Geometry check sheet. Reference: the model listing, model coordinates, mm. A direction names the side the tool comes from. Round coordinates to 2 decimals unless told otherwise and drop trailing zeros. Write item = value, one per line.
from build123d import *

# Parameters (mm, degrees)
SKETCH_1_R               = 1.75
EXTRUDE_1_DEPTH          = 6.6
EXTRUDE_1_2_DEPTH        = 6.6
SKETCH_2_R               = 50
EXTRUDE_2_DEPTH          = 3.4
SKETCH_4_R               = 1.75
CUT_EXTRUDE_2_DEPTH      = 10
SKETCH_5_R               = 36
EXTRUDE_3_DEPTH          = 4.3
EXTRUDE_4_DEPTH          = 30
SKETCH_9_R               = 10
EXTRUDE_6_DEPTH          = 10
SKETCH_10_R              = 50
CUT_EXTRUDE_4_DEPTH      = 14.3
CUT_EXTRUDE_7_DEPTH      = 20
SKETCH_13_W              = 36
SKETCH_13_H              = 160
CUT_EXTRUDE_8_DEPTH      = 10
SKETCH_14_R              = 3
CUT_EXTRUDE_9_DEPTH      = 10
CUT_EXTRUDE_START        = -10
CUT_EXTRUDE_10_DEPTH     = 10
SKETCH_16_R              = 3
CUT_EXTRUDE_11_DEPTH     = 10
PATTERN_CIRCULAR_1_COUNT = 5
PATTERN_CIRCULAR_1_ANGLE = 180
SKETCH_17_R              = 3
CUT_EXTRUDE_12_DEPTH     = 10
PATTERN_CIRCULAR_2_COUNT = 2
PATTERN_CIRCULAR_2_ANGLE = 45
PATTERN_CIRCULAR_3_COUNT = 2
PATTERN_CIRCULAR_3_ANGLE = 45
FILLET_1_R               = 2


# Read off the part's stored shape, not the designer's step: the extrude step
with BuildPart() as part:
    # Sketch 1 → Extrude 1 (new body)
    with BuildSketch(Plane.XY):
        with BuildLine():
            ThreePointArc((20.506096654, 20.506096654), (29, 0), (20.506096654, -20.506096654))
            Line((20.506096654, -20.506096654), (24.748737342, -24.748737342))
            ThreePointArc((24.748737342, -24.748737342), (24.748737342, -35.355339059), (35.355339059, -35.355339059))
            ThreePointArc((35.355339059, -35.355339059), (50, 0), (35.355339059, 35.355339059))
            ThreePointArc((35.355339059, 35.355339059), (24.748737342, 35.355339059), (24.748737342, 24.748737342))
            Line((24.748737342, 24.748737342), (20.506096654, 20.506096654))
        make_face()
        with Locations((30.0520382, 30.0520382)):
            Circle(SKETCH_1_R, mode=Mode.SUBTRACT)
        with Locations((30.0520382, -30.0520382)):
            Circle(SKETCH_1_R, mode=Mode.SUBTRACT)
        with Locations((42.5, 0)):
            Circle(SKETCH_1_R, mode=Mode.SUBTRACT)
    extrude(amount=EXTRUDE_1_DEPTH)



with BuildPart() as body_2:
    # Sketch 1 → Extrude 1 2 (new body)
    with BuildSketch(Plane.XY):
        with BuildLine():
            ThreePointArc((-35.355339059, 35.355339059), (-50, 0), (-35.355339059, -35.355339059))
            ThreePointArc((-35.355339059, -35.355339059), (-24.748737342, -35.355339059), (-24.748737342, -24.748737342))
            Line((-24.748737342, -24.748737342), (-20.506096654, -20.506096654))
            ThreePointArc((-20.506096654, -20.506096654), (-29, 0), (-20.506096654, 20.506096654))
            Line((-20.506096654, 20.506096654), (-24.748737342, 24.748737342))
            ThreePointArc((-24.748737342, 24.748737342), (-24.748737342, 35.355339059), (-35.355339059, 35.355339059))
        make_face()
        with Locations((-30.0520382, 30.0520382)):
            Circle(SKETCH_1_R, mode=Mode.SUBTRACT)
        with Locations((-30.0520382, -30.0520382)):
            Circle(SKETCH_1_R, mode=Mode.SUBTRACT)
        with Locations((-42.5, 0)):
            Circle(SKETCH_1_R, mode=Mode.SUBTRACT)
    extrude(amount=EXTRUDE_1_2_DEPTH)


with BuildPart() as part_1:
    add(part.part)

    add(body_2.part)  # Extrude 2 merges body 2
    # Sketch 2 → Extrude 2 (add)
    with BuildSketch(Plane.XY.offset(6.6)):
        with Locations(Location((0, 0, 0), (0, 0, 225))):
            Circle(SKETCH_2_R)
    extrude(amount=EXTRUDE_2_DEPTH)

    # Sketch 4 → Cut-Extrude 2 (cut, symmetric)
    with BuildSketch(Plane(origin=(0, 0, 6.6), x_dir=(-1, 0, 0), z_dir=(0, 0, -1))):
        with Locations(Location((-42.5, 0, 0), (0, 0, 180))):
            Circle(SKETCH_4_R)
        with Locations(Location((-30.0520382, 30.0520382, 0), (0, 0, 180))):
            Circle(SKETCH_4_R)
        with Locations(Location((-30.0520382, -30.0520382, 0), (0, 0, 180))):
            Circle(SKETCH_4_R)
        with Locations(Location((30.0520382, -30.0520382, 0), (0, 0, 180))):
            Circle(SKETCH_4_R)
        with Locations(Location((42.5, 0, 0), (0, 0, 180))):
            Circle(SKETCH_4_R)
        with Locations(Location((30.0520382, 30.0520382, 0), (0, 0, 180))):
            Circle(SKETCH_4_R)
    extrude(amount=CUT_EXTRUDE_2_DEPTH, both=True, mode=Mode.SUBTRACT)

    # Sketch 5 → Extrude 3 (add)
    with BuildSketch(Plane.XY.offset(10)):
        with Locations(Location((0, 0, 0), (0, 0, 180))):
            Circle(SKETCH_5_R)
    extrude(amount=EXTRUDE_3_DEPTH)

    # Sketch 8 → Extrude 4 (add)
    with BuildSketch(Plane.XY.offset(14.3)):
        with BuildLine():
            ThreePointArc((-6.785714286, -99.769504768), (100, 0), (-6.785714286, 99.769504768))
            ThreePointArc((-6.785714286, 99.769504768), (-245, 0), (-6.785714286, -99.769504768))
        make_face()
    extrude(amount=EXTRUDE_4_DEPTH)

    # Sketch 9 → Extrude 6 (add)
    with BuildSketch(Plane(origin=(0, 0, 14.3), x_dir=(-1, 0, 0), z_dir=(0, 0, -1))):
        with Locations(Location((105, 0, 0), (0, 0, 180))):
            Circle(SKETCH_9_R)
    extrude(amount=EXTRUDE_6_DEPTH)

    # Sketch 10 → Cut-Extrude 4 (cut)
    with BuildSketch(Plane(origin=(0, 0, 0), x_dir=(-1, 0, 0), z_dir=(0, 0, -1))):
        Circle(SKETCH_10_R)
    extrude(amount=-CUT_EXTRUDE_4_DEPTH, mode=Mode.SUBTRACT)

    # Sketch 11 → Cut-Extrude 7 (cut)
    with BuildSketch(Plane(origin=(0, 0, 14.3), x_dir=(-1, 0, 0), z_dir=(0, 0, -1))):
        Polygon((-18, -31.176914536), (18, -31.176914536), (36, 0), (18, 31.176914536), (-18, 31.176914536), (-36, 0), align=None)
    extrude(amount=-CUT_EXTRUDE_7_DEPTH, mode=Mode.SUBTRACT)

    # Sketch 13 → Cut-Extrude 8 (cut)
    with BuildSketch(Plane(origin=(0, 0, 14.3), x_dir=(-1, 0, 0), z_dir=(0, 0, -1))):
        Rectangle(SKETCH_13_W, SKETCH_13_H)
    extrude(amount=-CUT_EXTRUDE_8_DEPTH, mode=Mode.SUBTRACT)

    # Sketch 14 → Cut-Extrude 9 (cut)
    with BuildSketch(Plane(origin=(0, 0, 24.3), x_dir=(-1, 0, 0), z_dir=(0, 0, -1))):
        with Locations((0, 62)):
            Circle(SKETCH_14_R)
    cut_extrude_9 = extrude(amount=-CUT_EXTRUDE_9_DEPTH, mode=Mode.SUBTRACT)

    # Mirror 1: Cut-Extrude 9 across plane
    add(cut_extrude_9.mirror(Plane.ZX), mode=Mode.SUBTRACT)

    # Cut-Extrude 10 outline → Cut-Extrude 10 (cut)
    with BuildSketch(Plane(origin=(0, 0, 14.3), x_dir=(-1, 0, 0), z_dir=(0, 0, -1)).offset(CUT_EXTRUDE_START)):
        with BuildLine():
            ThreePointArc((213.166538264, 20), (215, 0), (213.166538264, -20.000000001))
            Line((213.166538264, -20.000000001), (215, -20))
            ThreePointArc((215, -20), (235.000000001, 0), (215, 20))
            Line((215, 20), (213.166538264, 20))
        make_face()
        with BuildLine():
            ThreePointArc((167.343157078, 90.627428329), (182.78174593, 77.781745931), (195.627428329, 62.343157079))
            Line((195.627428329, 62.343157079), (196.923881561, 63.63961031))
            ThreePointArc((196.923881561, 63.63961031), (196.923881554, 91.923881558), (168.639610306, 91.923881556))
            Line((168.639610306, 91.923881556), (167.343157078, 90.627428329))
        make_face()
        with BuildLine():
            ThreePointArc((195.627428318, -62.343157094), (182.781745927, -77.781745934), (167.343157087, -90.627428323))
            Line((167.343157087, -90.627428323), (168.639610312, -91.923881548))
            ThreePointArc((168.639610312, -91.923881548), (196.923881525, -91.923881572), (196.923881594, -63.639610359))
            Line((196.923881594, -63.639610359), (195.627428318, -62.343157094))
        make_face()
        with BuildLine():
            ThreePointArc((124.999999989, -108.166538266), (104.999999986, -110), (84.999999984, -108.166538261))
            Line((84.999999984, -108.166538261), (84.999999984, -109.999999998))
            ThreePointArc((84.999999984, -109.999999998), (104.999999924, -130.000000016), (125.000000016, -110.00000015))
            Line((125.000000016, -110.00000015), (124.999999989, -108.166538266))
        make_face()
        with BuildLine():
            ThreePointArc((85.00000001, 108.166538266), (105.000000014, 110), (125.000000017, 108.166538261))
            Line((125.000000017, 108.166538261), (124.999999989, 109.99999985))
            ThreePointArc((124.999999989, 109.99999985), (105.000000076, 129.999999989), (85.000000011, 110.000000002))
            Line((85.000000011, 110.000000002), (85.00000001, 108.166538266))
        make_face()
        with BuildLine():
            Line((-67.082039323, 20), (-70, 20))
            ThreePointArc((-70, 20), (-90, 0), (-70, -20))
            Line((-70, -20), (-67.082039323, -20))
            ThreePointArc((-67.082039323, -20), (-69.999999998, 0), (-67.082039323, 20))
        make_face()
        with BuildLine():
            ThreePointArc((-33.292029197, -61.576300568), (-49.497474649, -49.497474714), (-61.576300524, -33.292029278))
            Line((-61.576300524, -33.292029278), (-63.639610307, -35.355339059))
            ThreePointArc((-63.639610307, -35.355339059), (-63.6396103, -63.639610325), (-35.355339034, -63.639610318))
            Line((-35.355339034, -63.639610318), (-33.292029197, -61.576300568))
        make_face()
        with BuildLine():
            ThreePointArc((-61.576300517, 33.292029292), (-49.497474678, 49.497474685), (-33.292029283, 61.576300521))
            Line((-33.292029283, 61.576300521), (-35.355339063, 63.639610301))
            ThreePointArc((-35.355339063, 63.639610301), (-63.639610303, 63.639610311), (-63.639610293, 35.35533907))
            Line((-63.639610293, 35.35533907), (-61.576300517, 33.292029292))
        make_face()
    extrude(amount=CUT_EXTRUDE_10_DEPTH, mode=Mode.SUBTRACT)

    # Sketch 16 → Cut-Extrude 11 (cut)
    with BuildSketch(Plane(origin=(0, 0, 24.3), x_dir=(-1, 0, 0), z_dir=(0, 0, -1))):
        with Locations((104.999999997, 119.999999989)):
            Circle(SKETCH_16_R)
    cut_extrude_11 = extrude(amount=-CUT_EXTRUDE_11_DEPTH, mode=Mode.SUBTRACT)

    # Pattern Circular 1: Cut-Extrude 11 ×5 about axis
    pattern_circular_1_axis = Axis((-105, 0, 0), (0, 0, 1))
    for i in range(1, PATTERN_CIRCULAR_1_COUNT):
        add(cut_extrude_11.rotate(pattern_circular_1_axis, i * PATTERN_CIRCULAR_1_ANGLE / (PATTERN_CIRCULAR_1_COUNT - 1)), mode=Mode.SUBTRACT)

    # Sketch 17 → Cut-Extrude 12 (cut)
    with BuildSketch(Plane(origin=(0, 0, 24.3), x_dir=(-1, 0, 0), z_dir=(0, 0, -1))):
        with Locations((-80, 0)):
            Circle(SKETCH_17_R)
    cut_extrude_12 = extrude(amount=-CUT_EXTRUDE_12_DEPTH, mode=Mode.SUBTRACT)

    # Pattern Circular 2: Cut-Extrude 12 ×2 about axis
    pattern_circular_2_axis = Axis((0, 0, 34.3), (0, 0, 1))
    for i in range(1, PATTERN_CIRCULAR_2_COUNT):
        add(cut_extrude_12.rotate(pattern_circular_2_axis, i * PATTERN_CIRCULAR_2_ANGLE / (PATTERN_CIRCULAR_2_COUNT - 1)), mode=Mode.SUBTRACT)

    # Pattern Circular 3: Cut-Extrude 12 ×2 about axis
    pattern_circular_3_axis = Axis((0, 0, 34.3), (0, 0, -1))
    for i in range(1, PATTERN_CIRCULAR_3_COUNT):
        add(cut_extrude_12.rotate(pattern_circular_3_axis, i * PATTERN_CIRCULAR_3_ANGLE / (PATTERN_CIRCULAR_3_COUNT - 1)), mode=Mode.SUBTRACT)

    # Fillet 1
    fillet_1_edges = [part_1.edges().sort_by_distance(p)[0] for p in [
        (-245, 0, 14.3),
        (100, 0, 14.3),
        (-245, 0, 44.3),
        (100, 0, 44.3),
    ]]
    fillet(fillet_1_edges, radius=FILLET_1_R)


solid = part_1.part
(1) Tool access check on faces 1 (the flat face through (18, -56, 19)), 2 (the flat face through (-105, 0, 4.3)). Record the directions out of +Z, -Z, +X, -X, +Y, -Y that give a thin tool (end or side, any length) a straight path to the whole face; none if there is none.
Result set:
face_1 = -Z
face_2 = -Z, +X, -X, +Y, -Y
(2) Material ranges on line 1 along Y through (x, z) = (0, 27); line 2 along Y through (x, z) = (-105, 30.25); line 3 along Y through (x, z) = (-110.5, 17.5), recorded low to high. Write a range as from..to.
Result set:
line_1 = -100..-65, -59..-31.18, 31.18..59, 65..100
line_2 = -140..-123, -117..117, 123..140
line_3 = -139.89..-129.23, -109.86..109.86, 129.23..139.89
(3) Depth check by flat-ended pin: pin 1 Ø6.5 at (x, y) = (-225.5, 0) entering from -Z; pin 2 Ø1 at (x, z) = (-168.5, 34.5) entering from +Y; pin 3 Ø5 at (x, y) = (80, 0) entering from -Z. Enter the tip coordinate at first touch or a pass-through.
Result set:
pin_1 = 24.3
pin_2 = 125.02
pin_3 = 34.3
(4) Release check for a two-part mould opening along Y. For faces 3 (the cylindrical face through (-105, -110, 19)), 4 (the cylindrical face through (-244.924, 4.602, 29.118)), 5 (the flat face through (-75, 2, 14.3)) record: released by +Y, released by -Y, zero draft, split by the parting line, or undercut.
Result set:
face_3 = undercut
face_4 = split by the parting line
face_5 = zero draft
